from build123d import *

# Parameters (mm, degrees)
SKETCH1_R           = 75
BOSS_EXTRUDE1_DEPTH = 2.9
SKETCH2_W           = 70
SKETCH2_H           = 6
SKETCH2_R           = 1.4
CUT_EXTRUDE1_DEPTH  = 10
SKETCH3_R           = 1.7
CUT_EXTRUDE3_DEPTH  = 10


with BuildPart() as part:
    # Sketch1 → Boss-Extrude1 (new body)
    with BuildSketch(Plane(origin=(0, 0, 0), x_dir=(1, 0, 0), z_dir=(0, 1, 0))):
        with Locations(Location((0, 0, 0), (0, 0, 270))):
            Circle(SKETCH1_R)
    extrude(amount=BOSS_EXTRUDE1_DEPTH)

    # Sketch2 → Cut-Extrude1 (cut)
    with BuildSketch(Plane(origin=(0, 2.9, 0), x_dir=(1, 0, 0), z_dir=(0, 1, 0))):
        with Locations((0, -58.709242105)):
            Rectangle(SKETCH2_W, SKETCH2_H)
        with Locations((0, 58.709242105)):
            Rectangle(SKETCH2_W, SKETCH2_H)
        with BuildLine():
            ThreePointArc((-68.72850121, -30.023209712), (-54.08520342, 0), (-68.72850121, 30.023209712))
            ThreePointArc((-68.72850121, 30.023209712), (-75, 0), (-68.72850121, -30.023209712))
        make_face()
        with BuildLine():
            ThreePointArc((68.72850121, -30.023209712), (75, 0), (68.72850121, 30.023209712))
            ThreePointArc((68.72850121, 30.023209712), (54.08520342, 0), (68.72850121, -30.023209712))
        make_face()
        with Locations(Location((-22.14, -46.709242105, 0), (0, 0, 270))):
            Circle(SKETCH2_R)
        with Locations(Location((-2.56, -46.709242105, 0), (0, 0, 270))):
            Circle(SKETCH2_R)
        with Locations(Location((22.14, 46.709242105, 0), (0, 0, 270))):
            Circle(SKETCH2_R)
        with Locations(Location((2.56, 46.709242105, 0), (0, 0, 270))):
            Circle(SKETCH2_R)
    extrude(amount=-CUT_EXTRUDE1_DEPTH, mode=Mode.SUBTRACT)

    # Sketch3 → Cut-Extrude3 (cut)
    with BuildSketch(Plane(origin=(0, 2.9, 0), x_dir=(1, 0, 0), z_dir=(0, 1, 0))):
        with Locations(Location((-26.78520342, 5.5, 0), (0, 0, 270))):
            Circle(SKETCH3_R)
        with Locations(Location((-14.08520342, -5.6, 0), (0, 0, 270))):
            Circle(SKETCH3_R)
        with BuildLine():
            Line((-51.177473943, 2.65), (-54.177473943, 2.65))
            ThreePointArc((-54.177473943, 2.65), (-54.08520342, 0), (-54.177473943, -2.65))
            Line((-54.177473943, -2.65), (-51.177473943, -2.65))
            Line((-51.177473943, -2.65), (-51.177473943, 2.65))
        make_face()
    extrude(amount=-CUT_EXTRUDE3_DEPTH, mode=Mode.SUBTRACT)


solid = part.part
CAD build for the part. Positions are in the model's coordinates, mm. A direction names the side the tool comes from. Round coordinates to 2 decimals unless told otherwise and drop trailing zeros. Loops run counter-clockwise (first coordinate to the right, second up) from the corner with the lowest first, then second, coordinate; pieces in that order, holes last.
(1) Two-plate mould, pull along Z, no slides. Class faces 3 (the cylindrical face through (-1.22, 1.43, 74.99)), 4 (the cylindrical face through (-58.44, 1.47, -17.69)), 5 (the cylindrical face through (1.22, 1.43, -74.99)): +Z half, -Z half, draft (parallel to the pull), parting line (faces both ways), or undercut.
(2) Which spindle directions (+Z, -Z, +X, -X, +Y, -Y) get a long thin tool onto all of the face, cutting with end or side? Do faces 1 (the cylindrical face through (-15.745, 1.47, 5.231)), 2 (the cylindrical face through (-58.65, 1.47, 18.08)). Say none if no direction does.
(3) Cut at C-C (y = 1.5). State how many separate pieces and enclosed holes the cut face has, plus the area to 3 significant figures.
(4) Cut at D-D (z = -36.5). Give the cut face in (x, y).
(5) Cut at A-A (x = -7.5). Give the cut face in (y, z), plus the area to 3 significant figures.
(6) Drop flat-ended pins along their axis: pin 1 (2.5 mm diameter, centred on x = 22.14, z = -46.71, fed in from +Y); pin 2 (1.4 mm diameter, centred on y = 2, z = 0, fed in from -X); pin 3 (1.5 mm diameter, centred on y = 1.5, z = 36.5, fed in from +X); pin 4 (0.9 mm diameter, centred on x = -52.5, y = 1.5, fed in from +Z). Give the stop position or say it passes through.
(7) Cut at B-B (z = 5.6). Give the cut face in (x, y).
(8) Wall check: line 1 along Z through (x, y) = (-8.5, 1.1); line 2 along Z through (x, y) = (-16, 0.9); line 3 along X through (y, z) = (1.5, 5.6). Give the ranges that are in metal, low to high.
Findings below:
1. face 3: +Z half
1. face 4: undercut
1. face 5: -Z half
2. face 1: +Y, -Y
2. face 2: -X, +Y, -Y
3. separate pieces: 1
3. enclosed holes: 8
3. area: 15,000 mm2
4. outline: (-65.52, 0) - (65.52, 0) - (65.52, 2.9) - (-65.52, 2.9) - close
5. outline: (0, -74.62) - (2.9, -74.62) - (2.9, -61.71) - (0, -61.71) - close; (0, -55.71) - (2.9, -55.71) - (2.9, 55.71) - (0, 55.71) - close; (0, 61.71) - (2.9, 61.71) - (2.9, 74.62) - (0, 74.62) - close
5. area: 398 mm2
6. pin 1: passes through
6. pin 2: stops at x = -51.18
6. pin 3: stops at x = 65.93
6. pin 4: stops at z = 54
7. outline: (-54.5, 0) - (-15.79, 0) - (-15.79, 2.9) - (-54.5, 2.9) - close; (-12.39, 0) - (54.5, 0) - (54.5, 2.9) - (-12.39, 2.9) - close
8. line 1: z = -74.52 to -61.71, -55.71 to 55.71, 61.71 to 74.52
8. line 2: z = -73.27 to -61.71, -55.71 to 55.71, 61.71 to 73.27
8. line 3: x = -54.5 to -15.79, -12.39 to 54.5
